Read the model definition and answer for the solid it produces. Units are mm, in the model's axes. A direction names the side the tool comes from. Give positions to 0.01 mm unless a question says otherwise; leave off trailing zeros. Write each loop counter-clockwise with the first axis right and the second up, starting at its lowest first coordinate (ties: lowest second). Pieces come first, ordered by that corner, then holes. Notation, with made-up numbers: M -20.75,-34.5 L 14.25,-34.5 A22 cw 14.25,-13.5 Z; hole C 54.25,-34 d3. An arc over 180 degrees is marked long. Answer as CSV lines item,"result". Start each with the question number.
```python
from build123d import *

# Parameters (mm, degrees)
SKETCH_1_W          = 370
SKETCH_1_H          = 400
EXTRUDE_1_DEPTH     = 132
SKETCH_2_W          = 12
SKETCH_2_H          = 119.999999988
CUT_EXTRUDE_1_DEPTH = 449.273354104
SKETCH_3_W          = 400
SKETCH_3_H          = 100
EXTRUDE_2_DEPTH     = 77
SKETCH_4_W          = 12
SKETCH_4_H          = 119.999999988
CUT_EXTRUDE_2_DEPTH = 479.773432847
SKETCH_5_W          = 400
SKETCH_5_H          = 100
EXTRUDE_3_DEPTH     = 77
CUT_EXTRUDE_3_DEPTH = 479.773432847
HOLE_WIZARD_1_D     = 100
FILLET_1_R          = 50


with BuildPart() as part:
    # 草图1 → 凸台-拉伸1 (new body)
    with BuildSketch(Plane.XZ.offset(82)):
        Rectangle(SKETCH_1_W, SKETCH_1_H)
    extrude(amount=-EXTRUDE_1_DEPTH)

    # 草图2 → 切除-拉伸1 (cut, through all)
    with BuildSketch(Plane.XY.offset(200)):
        with Locations((-179, -9.999999994)):
            Rectangle(SKETCH_2_W, SKETCH_2_H)
    extrude(amount=-CUT_EXTRUDE_1_DEPTH, mode=Mode.SUBTRACT)

    # 草图3 → 凸台-拉伸2 (add)
    with BuildSketch(Plane.ZY.offset(173)):
        Rectangle(SKETCH_3_W, SKETCH_3_H)
    extrude(amount=EXTRUDE_2_DEPTH)

    # 草图4 → 切除-拉伸2 (cut, through all)
    with BuildSketch(Plane.XY.offset(200)):
        with Locations((179, -9.999999994)):
            Rectangle(SKETCH_4_W, SKETCH_4_H)
    extrude(amount=-CUT_EXTRUDE_2_DEPTH, mode=Mode.SUBTRACT)

    # 草图5 → 凸台-拉伸3 (add)
    with BuildSketch(Plane(origin=(173, 0, 0), x_dir=(0, 0, -1), z_dir=(1, 0, 0))):
        Rectangle(SKETCH_5_W, SKETCH_5_H)
    extrude(amount=EXTRUDE_3_DEPTH)

    # 草图6 → 切除-拉伸3 (cut, through all)
    with BuildSketch(Plane(origin=(0, 0, -200), x_dir=(-1, 0, 0), z_dir=(0, 0, -1))):
        Polygon((-137, -82), (137, -82), (137, -69.999999997), (149, -69.999999997), (149, -50), (-149, -50), (-149, -69.999999997), (-137, -69.999999997), align=None)
    extrude(amount=-CUT_EXTRUDE_3_DEPTH, mode=Mode.SUBTRACT)

    # 孔1 (through all)
    with Locations(Plane(origin=(0, -50, 0), x_dir=(-1, 0, 0), z_dir=(0, -1, 0))):
        with Locations((0, 0)):
            Hole(HOLE_WIZARD_1_D / 2)

    # 圆角1
    fillet_1_edges = [part.edges().sort_by_distance(p)[0] for p in [
        (-250, 0, -200),
        (-250, 0, 200),
        (250, 0, -200),
        (250, 0, 200),
    ]]
    fillet(fillet_1_edges, radius=FILLET_1_R)


solid = part.part
```
1. Find section A-A on x = 0. Determine the outline of the cut face in (y, z), then the cut area to 3 significant figures.
2. For faces 5 (the face through (-3, -2, 200)), 6 (the face through (179, -70, 3)), 7 (the face through (149, -60, -3)), 8 (the face through (-179, -70, 3)), 9 (the face through (137, -76, -3)), determine the directions among +Z, -Z, +X, -X, +Y, -Y from which every point of the face is accessible in a straight line to the end or side of a thin tool.
3. Given pin 1 (9.5 mm diameter, centred on y = -74.5, z = 68, fed in from +X); pin 2 (1.5 mm diameter, centred on y = -58.5, z = 122.5, fed in from -X); pin 3 (13 mm diameter, centred on y = -77.5, z = 52, fed in from -X), each flat-ended and moving along its own axis, determine where each tip first touches the part or whether it passes through.
4. Find section D-D on z = -123. Determine the outline of the cut face in (x, y), then the cut area to 3 significant figures.
5. Find the intervals of material crossed by line 1 (Z direction, x = 0, y = 9); line 2 (Y direction, x = -141, z = -148.5); line 3 (X direction, y = -65, z = 68), in increasing order. Write a range as [from, to].
6. Find section B-B on z = 0. Determine the outline of the cut face in (x, y), then the cut area to 3 significant figures.
7. Find section C-C on y = 19.5. Determine the outline of the cut face in (x, z).
8. Determine the mould class of faces 1 (the face through (143, -70, -3)), 2 (the face through (-143, -70, -3)), 3 (the face through (185, -76, -3)), 4 (the face through (161, -82, 3)) for opening direction Y: +Y half, -Y half, draft (parallel to the pull), parting line (faces both ways), or undercut.
Computed:
1,outline,"M -50,-200 L 50,-200 L 50,-50 L -50,-50 Z; M -50,50 L 50,50 L 50,200 L -50,200 Z"
1,area,"30,000 mm^2"
2,face 5,"+Z, +X, -X, +Y, -Y"
2,face 6,"+Z, -Z, +X"
2,face 7,"+Z, -Z"
2,face 8,"+Z, -Z, -X"
2,face 9,"+Z, -Z, -Y"
3,pin 1,"stops at x = 185"
3,pin 2,"stops at x = -173"
3,pin 3,"stops at x = -185"
4,outline,"M -250,-50 L -173,-50 L -173,-70 L -185,-70 L -185,-82 L -137,-82 L -137,-70 L -149,-70 L -149,-50 L 149,-50 L 149,-70 L 137,-70 L 137,-82 L 185,-82 L 185,-70 L 173,-70 L 173,-50 L 250,-50 L 250,50 L -250,50 Z"
4,area,"52,100 mm^2"
5,line 1,"z = [-200, -50], [50, 200]"
5,line 2,"y = [-82, -70], [-50, 50]"
5,line 3,"x = [-173, -149], [149, 173]"
6,outline,"M -250,-50 L -173,-50 L -173,-70 L -185,-70 L -185,-82 L -137,-82 L -137,-70 L -149,-70 L -149,-50 L -50,-50 L -50,50 L -250,50 Z; M 50,-50 L 149,-50 L 149,-70 L 137,-70 L 137,-82 L 185,-82 L 185,-70 L 173,-70 L 173,-50 L 250,-50 L 250,50 L 50,50 Z"
6,area,"42,100 mm^2"
7,outline,"M -250,-150 A50 ccw -200,-200 L 200,-200 A50 ccw 250,-150 L 250,150 A50 ccw 200,200 L -200,200 A50 ccw -250,150 Z; hole C 0,0 d100"
8,face 1,"undercut"
8,face 2,"undercut"
8,face 3,"draft"
8,face 4,"-Y half"
